from build123d import *

# Parameters (mm, degrees)
SKETCH1_W             = 180
SKETCH1_H             = 90
BOSS_EXTRUDE1_DEPTH   = 5
F_1_0MM_DOWEL_HOLE1_D = 8


with BuildPart() as part:
    # Sketch1 → Boss-Extrude1 (new body)
    with BuildSketch(Plane(origin=(0, 0, 0), x_dir=(1, 0, 0), z_dir=(0, 1, 0))):
        Rectangle(SKETCH1_W, SKETCH1_H)
    extrude(amount=BOSS_EXTRUDE1_DEPTH)

    # Ø1.0mm Dowel Hole1 (through all)
    with Locations(Plane(origin=(0, 5, 0), x_dir=(1, 0, 0), z_dir=(0, 1, 0))):
        with Locations((-77, 20), (-77, -15), (-30, -32), (30, -32), (77, -15), (77, 20)):
            Hole(F_1_0MM_DOWEL_HOLE1_D / 2)


solid = part.part
Input: part model. Units: mm. Frame: model coordinates. Round coordinates to 2 decimals unless told otherwise and drop trailing zeros. Loops run counter-clockwise (first coordinate to the right, second up) from the corner with the lowest first, then second, coordinate; pieces in that order, holes last. Notation, with made-up numbers: M 22,-16.75 L 71,-16.75 A18 cw 71,8.25 Z; hole C 44.25,80 d11. An arc over 180 degrees is marked long. Answer as CSV lines item,"result". Start each with the question number.
(1) Line query: line 1 (Z direction, x = -77, y = 2.1); line 2 (X direction, y = 1, z = -20); line 3 (Z direction, x = -30, y = 4). Output: solid intervals per line, ascending. Write a range as [from, to].
(2) Draft query along X for faces 1 (the cylindrical face through (30.521, 2.465, 28.034)), 2 (the cylindrical face through (-74.05, 2.47, 12.3)), 3 (the flat face through (-1, 5, -1)), 4 (the flat face through (-90, 2, 1)). Return one class per face: released by +X, released by -X, zero draft, split by the parting line, or undercut.
(3) Section A-A, the plane z = 32. Output: boundary loops of the cut face in (x, y).
(4) Section C-C, the plane x = 30. Output: boundary loops of the cut face in (y, z), plus the area to 3 significant figures.
(5) Section B-B, the plane x = 77. Output: boundary loops of the cut face in (y, z).
(6) Section D-D, the plane y = 0.8. Output: boundary loops of the cut face in (x, z), plus the area to 3 significant figures.
Values found:
1,line 1,"z = [-45, -24], [-16, 11], [19, 45]"
1,line 2,"x = [-90, -81], [-73, 73], [81, 90]"
1,line 3,"z = [-45, 28], [36, 45]"
2,face 1,"undercut"
2,face 2,"undercut"
2,face 3,"zero draft"
2,face 4,"released by -X"
3,outline,"M -90,0 L -34,0 L -34,5 L -90,5 Z; M -26,0 L 26,0 L 26,5 L -26,5 Z; M 34,0 L 90,0 L 90,5 L 34,5 Z"
4,outline,"M 0,-45 L 5,-45 L 5,28 L 0,28 Z; M 0,36 L 5,36 L 5,45 L 0,45 Z"
4,area,"410 mm²"
5,outline,"M 0,-45 L 5,-45 L 5,-24 L 0,-24 Z; M 0,-16 L 5,-16 L 5,11 L 0,11 Z; M 0,19 L 5,19 L 5,45 L 0,45 Z"
6,outline,"M -90,-45 L 90,-45 L 90,45 L -90,45 Z; hole C -77,-20 d8; hole C -77,15 d8; hole C -30,32 d8; hole C 30,32 d8; hole C 77,-20 d8; hole C 77,15 d8"
6,area,"15,900 mm²"
